```python
from build123d import *

# Parameters (mm, degrees)
BOSS_EXTRUDE1_DEPTH     = 30
SKETCH1_13_W            = 0.5
SKETCH1_13_H            = 10.5
BOSS_EXTRUDE6_DEPTH     = 30
CUT_EXTRUDE3_DEPTH      = 5
BOSS_EXTRUDE4_START     = -2.45
BOSS_EXTRUDE4_OUTLINE_R = 1.6
BOSS_EXTRUDE4_DEPTH     = 2.45
CUT_EXTRUDE1_DEPTH      = 5
SKETCH1_10_R            = 1.6
BOSS_EXTRUDE5_DEPTH     = 2.45
CUT_EXTRUDE4_DEPTH      = 63.283625457


# Read off the part's stored shape, not the designer's step: Boss-Extrude4
with BuildPart() as part:
    # Sketch1 → Boss-Extrude1 (new body)
    with BuildSketch(Plane.XY):
        Polygon((13, 0), (0, 10.5), (0, 0), align=None)
    boss_extrude1 = extrude(amount=BOSS_EXTRUDE1_DEPTH)

    # Sketch1<13> → Boss-Extrude6 (add)
    with BuildSketch(Plane.XY):
        with Locations((-0.25, 5.25)):
            Rectangle(SKETCH1_13_W, SKETCH1_13_H)
    boss_extrude6 = extrude(amount=BOSS_EXTRUDE6_DEPTH)

    # Sketch4 → Cut-Extrude3 (cut)
    with BuildSketch(Plane(origin=(5.132497762, 6.354521038, 0), x_dir=(0, 0, -1), z_dir=(0.6283371070876215, 0.7779411802037215, 0))):
        Polygon((-11.825, -10.113235343), (-6.175, -10.113235343), (-6.175, 0.645733136), (-9, 2.276747647), (-11.825, 0.645733136), align=None)
    cut_extrude3 = extrude(amount=-CUT_EXTRUDE3_DEPTH, mode=Mode.SUBTRACT)

    # Boss-Extrude4 outline → Boss-Extrude4 (add)
    with BuildSketch(Plane(origin=(5.132497762, 6.354521038, 0), x_dir=(0, 0, -1), z_dir=(0.6283371070876215, 0.7779411802037215, 0)).offset(BOSS_EXTRUDE4_START)):
        Polygon((-6.175, -0.985281374), (0, -0.985281374), (0, 3.886764657), (-30, 3.886764657), (-30, -10.113235343), (0, -10.113235343), (0, -8.485281374), (-6.175, -8.485281374), align=None)
        with Locations((-9, -0.985281374)):
            Circle(BOSS_EXTRUDE4_OUTLINE_R, mode=Mode.SUBTRACT)
    boss_extrude4 = extrude(amount=BOSS_EXTRUDE4_DEPTH)

    # Sketch1<4> → Cut-Extrude1 (cut)
    with BuildSketch(Plane.XY):
        Polygon((9.15, 0), (9.15, 2.387149176), (3.906218974, 6.622510773), (0.862333294, 5.449653878), (0.356114319, 2.227143105), (3.113529592, 0), align=None)
    cut_extrude1 = extrude(amount=CUT_EXTRUDE1_DEPTH, mode=Mode.SUBTRACT)

    # Sketch1<10> → Boss-Extrude5 (add)
    with BuildSketch(Plane.XY):
        Polygon((3.113529592, 0), (9.15, 0), (9.15, 2.387149176), (3.906218974, 6.622510773), (0.862333294, 5.449653878), (0.356114319, 2.227143105), align=None)
        with Locations((3.4, 3.4)):
            Circle(SKETCH1_10_R, mode=Mode.SUBTRACT)
    boss_extrude5 = extrude(amount=BOSS_EXTRUDE5_DEPTH)

    # Mirror1: Boss-Extrude1, Boss-Extrude6, Cut-Extrude3, Boss-Extrude4, Cut-Extrude1, Boss-Extrude5 across plane
    add(boss_extrude1.mirror(Plane.XY.offset(30)))
    add(boss_extrude6.mirror(Plane.XY.offset(30)))
    add(cut_extrude3.mirror(Plane.XY.offset(30)), mode=Mode.SUBTRACT)
    add(boss_extrude4.mirror(Plane.XY.offset(30)))
    add(cut_extrude1.mirror(Plane.XY.offset(30)), mode=Mode.SUBTRACT)
    add(boss_extrude5.mirror(Plane.XY.offset(30)))

    # Sketch1<12> → Cut-Extrude4 (cut, through all)
    with BuildSketch(Plane.XY):
        Polygon((13, -3.5), (13, 0), (12.105518027, 0), (9.15, 0), (3.4, 0), (3.113529592, 0), (0, 0), (0, -3.5), align=None)
    extrude(amount=CUT_EXTRUDE4_DEPTH, mode=Mode.SUBTRACT)


solid = part.part
```
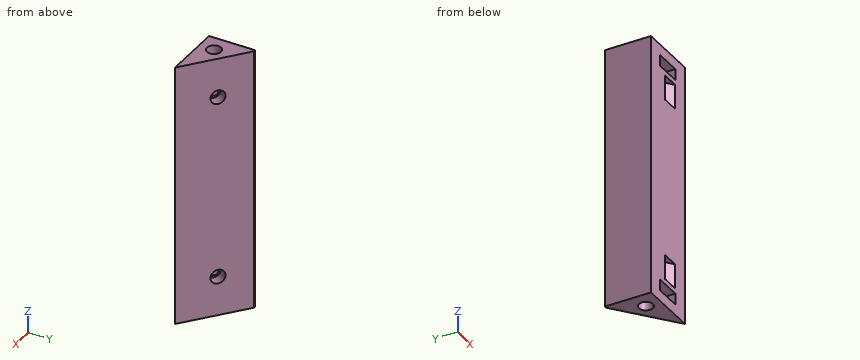
Geometry check sheet. Reference: the model listing, model coordinates, mm. Coordinates: 2 decimals unless noted, no trailing zeros. Loops run counter-clockwise (first coordinate to the right, second up) from the corner with the lowest first, then second, coordinate; pieces in that order, holes last. Notation, with made-up numbers: (-1.75, 76.5) - (51.25, 76.5) arc R20 cw to (51.25, 104.5) - close; hole circle Ø1 at (-6, 76.5). An arc over 180 degrees is marked (long way). One line per item, written item: value. Start each with the question number.
(1) Cross-section at B-B on z = 23. Enter the section's corners in (x, y), plus the area to 3 significant figures.
(2) Depth check by flat-ended pin: P1, Ø3.5, axis at x = 3.4, y = 3.4, coming from the -Z side; P2, Ø2, axis at y = 3, z = 19, coming from the +X side; P3, Ø2, axis at x = 11.5, y = 4.5, coming from the -Z side; P4, Ø3, axis at y = 6.5, z = 22.5, coming from the +X side. Enter the tip coordinate at first touch or a pass-through.
(3) Cross-section at A-A on x = 8. Enter the section's corners in (y, z) (3 decimals), plus the area to 3 significant figures.
(4) Material ranges on line 1 (Y direction, x = 7, z = 22); line 2 (Y direction, x = 3.4, z = 58.6); line 3 (Z direction, x = 4.25, y = 5), recorded low to high. Write a range as [from, to].
(5) Cross-section at C-C on y = 9.75. Enter the section's corners in (x, z).
Results below:
1. outline: (-0.5, 0) - (13, 0) - (0, 10.5) - (-0.5, 10.5) - close
1. area: 73.5 mm2
2. P1: stops at z = 0
2. P2: stops at x = 10.52
2. P3: passes through
2. P4: stops at x = 6.81
3. outline: (0, 0) - (4.038, 0) - (4.038, 60) - (0, 60) - (0, 57.55) - (3.316, 57.55) - (3.316, 55) - (0, 55) - (0, 53.825) - (0.889, 53.825) - (0.889, 48.175) - (0, 48.175) - (0, 11.825) - (0.889, 11.825) - (0.889, 6.175) - (0, 6.175) - (0, 5) - (3.316, 5) - (3.316, 2.45) - (0, 2.45) - close
3. area: 215 mm2
4. line 1: y = [0, 4.85]
4. line 2: y = [0, 1.8], [5, 7.75]
4. line 3: z = [0, 2.45], [5, 7.63], [10.37, 49.63], [52.37, 55], [57.55, 60]
5. outline: (-0.5, 0) - (0.93, 0) - (0.93, 60) - (-0.5, 60) - close
